from build123d import *

# Parameters (mm, degrees)
SKETCH1_W           = 38.1
SKETCH1_H           = 63.5
SKETCH1_W_2         = 25.4
SKETCH1_H_2         = 50.8
BOSS_EXTRUDE1_DEPTH = 50.8
SKETCH4_W           = 25.4
SKETCH4_H           = 5.461
SKETCH4_W_2         = 2.921
SKETCH4_H_2         = 39.878
BOSS_EXTRUDE2_DEPTH = 2.54
SKETCH5_W           = 2.921
SKETCH5_H           = 50.8
BOSS_EXTRUDE3_DEPTH = 5.588
SKETCH6_W           = 2.54
SKETCH6_H           = 5.461
CUT_EXTRUDE1_DEPTH  = 2.54


with BuildPart() as part:
    # Sketch1 → Boss-Extrude1 (new body)
    with BuildSketch(Plane.XY):
        with Locations((4.108271787, -2.227658789)):
            Rectangle(SKETCH1_W, SKETCH1_H)
        with Locations((4.108271787, -2.227658789)):
            Rectangle(SKETCH1_W_2, SKETCH1_H_2, mode=Mode.SUBTRACT)
    extrude(amount=BOSS_EXTRUDE1_DEPTH)

    # Sketch4 → Boss-Extrude2 (add)
    with BuildSketch(Plane(origin=(0, 0, 5.588), x_dir=(-1, 0, 0), z_dir=(0, 0, -1))):
        with Locations((-4.108271787, 20.441841211)):
            Rectangle(SKETCH4_W, SKETCH4_H)
        with Locations((-15.347771787, -2.227658789)):
            Rectangle(SKETCH4_W_2, SKETCH4_H_2)
        with Locations((-4.108271787, -24.897158789)):
            Rectangle(SKETCH4_W, SKETCH4_H)
        with Locations((7.131228213, -2.227658789)):
            Rectangle(SKETCH4_W_2, SKETCH4_H_2)
    extrude(amount=-BOSS_EXTRUDE2_DEPTH)

    # Sketch5 → Boss-Extrude3 (add)
    with BuildSketch(Plane(origin=(0, 0, 5.588), x_dir=(-1, 0, 0), z_dir=(0, 0, -1))):
        with Locations((-15.347771787, -2.227658789)):
            Rectangle(SKETCH5_W, SKETCH5_H)
        with Locations((7.131228213, -2.227658789)):
            Rectangle(SKETCH5_W, SKETCH5_H)
    extrude(amount=BOSS_EXTRUDE3_DEPTH)

    # Sketch6 → Cut-Extrude1 (cut)
    with BuildSketch(Plane(origin=(0, 0, 5.588), x_dir=(-1, 0, 0), z_dir=(0, 0, -1))):
        with Locations((-4.108271787, 20.441841211)):
            Rectangle(SKETCH6_W, SKETCH6_H)
        with Locations((-4.108271787, -24.897158789)):
            Rectangle(SKETCH6_W, SKETCH6_H)
    extrude(amount=-CUT_EXTRUDE1_DEPTH, mode=Mode.SUBTRACT)


solid = part.part
Model file for the job. Use its own axes, mm. A direction names the side the tool comes from. Round coordinates to 2 decimals unless told otherwise and drop trailing zeros. Loops run counter-clockwise (first coordinate to the right, second up) from the corner with the lowest first, then second, coordinate; pieces in that order, holes last. Notation, with made-up numbers: (50.25, -32) -> (90.25, -32) arc R18 cw to (90.25, -17) -> close; hole circle Ø10 at (7, 12.5). An arc over 180 degrees is marked (long way). Answer as CSV lines item,"result". Start each with the question number.
1) Pin check, flat tips, straight feed: P1, Ø12.5, axis at x = -5, y = -7.5, coming from the +Z side; P2, Ø5.5, axis at x = 13, y = 1, coming from the +Z side; P3, Ø2.5, axis at x = 10.5, y = 20, coming from the -Z side. Stop position of each tip, or through.
2) Tool access for faces 1 (the face through (-1, -22.167, 7)), 2 (the face through (10, -25, 5.588)), 3 (the face through (23.158, -3, 25)), 4 (the face through (15, -2, 8.128)): list every direction of +Z, -Z, +X, -X, +Y, -Y with a clear straight run to the whole face (end or side of a thin tool).
3) Slice it at A-A (x = 4). List the corners of the cut face in (y, z).
4) Slice it at D-D (x = 15). List the corners of the cut face in (y, z), plus the area to 3 significant figures.
5) Slice it at C-C (z = 3.5). List the corners of the cut face in (x, y).
6) Slice it at B-B (z = 24.5). List the corners of the cut face in (x, y), plus the area to 3 significant figures.
7) Mould opens along Y. For faces 5 (the face through (17, -2, 0)), 6 (the face through (13.887, -3, 4)), 7 (the face through (-1, -25, 5.588)) say: +Y half, -Y half, draft (parallel to the pull), parting line (faces both ways), or undercut.
8) Probe line 1 along X through (y, z) = (14.5, 34.5); line 2 along Y through (x, z) = (10, 36); line 3 along X through (y, z) = (20, 4). List the from-to ranges inside material, lowest first.
Filled in:
1,P1,"stops at z = 50.8"
1,P2,"stops at z = 8.13"
1,P3,"stops at z = 5.59"
2,face 1,"+Z, -Z"
2,face 2,"-Z"
2,face 3,"+Z, -Z, +X, +Y, -Y"
2,face 4,"+Z"
3,outline,"(-33.98, 0) -> (-27.63, 0) -> (-27.63, 50.8) -> (-33.98, 50.8) -> close; (23.17, 0) -> (29.52, 0) -> (29.52, 50.8) -> (23.17, 50.8) -> close"
4,outline,"(-33.98, 0) -> (29.52, 0) -> (29.52, 50.8) -> (23.17, 50.8) -> (23.17, 8.13) -> (-27.63, 8.13) -> (-27.63, 50.8) -> (-33.98, 50.8) -> close"
4,area,"1,060 mm2"
5,outline,"(-14.94, -33.98) -> (23.16, -33.98) -> (23.16, 29.52) -> (-14.94, 29.52) -> close; hole (-5.67, -27.63) -> (13.89, -27.63) -> (13.89, 23.17) -> (-5.67, 23.17) -> close"
6,outline,"(-14.94, -33.98) -> (23.16, -33.98) -> (23.16, 29.52) -> (-14.94, 29.52) -> close; hole (-8.59, -27.63) -> (16.81, -27.63) -> (16.81, 23.17) -> (-8.59, 23.17) -> close"
6,area,"1,130 mm2"
7,face 5,"draft"
7,face 6,"undercut"
7,face 7,"undercut"
8,line 1,"x = -14.94 to -8.59, 16.81 to 23.16"
8,line 2,"y = -33.98 to -27.63, 23.17 to 29.52"
8,line 3,"x = -14.94 to -5.67, 13.89 to 23.16"
